```python
from build123d import *

# Parameters (mm, degrees)
SKETCH1_W           = 50.8
SKETCH1_H           = 25.4
SKETCH1_W_2         = 44.45
SKETCH1_H_2         = 19.05
BOSS_EXTRUDE1_DEPTH = 254
SKETCH2_R           = 14.2875
CUT_EXTRUDE1_DEPTH  = 26.4
SKETCH3_R           = 3.175
CUT_EXTRUDE2_DEPTH  = 26.4
CUT_EXTRUDE3_DEPTH  = 26.4


with BuildPart() as part:
    # Sketch1 → Boss-Extrude1 (new body)
    with BuildSketch(Plane.XY):
        with Locations((25.4, 12.7)):
            Rectangle(SKETCH1_W, SKETCH1_H)
        with Locations((25.4, 12.7)):
            Rectangle(SKETCH1_W_2, SKETCH1_H_2, mode=Mode.SUBTRACT)
    extrude(amount=BOSS_EXTRUDE1_DEPTH)

    # Sketch2 → Cut-Extrude1 (cut, through all)
    with BuildSketch(Plane(origin=(0, 25.4, 0), x_dir=(1, 0, 0), z_dir=(0, 1, 0))):
        with Locations((31.75, -19.05)):
            Circle(SKETCH2_R)
        with Locations((31.75, -171.45)):
            Circle(SKETCH2_R)
    extrude(amount=-CUT_EXTRUDE1_DEPTH, mode=Mode.SUBTRACT)

    # Sketch3 → Cut-Extrude2 (cut, through all)
    with BuildSketch(Plane(origin=(0, 25.4, 0), x_dir=(1, 0, 0), z_dir=(0, 1, 0))):
        with Locations((25.4, -244.475)):
            Circle(SKETCH3_R)
    extrude(amount=-CUT_EXTRUDE2_DEPTH, mode=Mode.SUBTRACT)

    # Sketch4 → Cut-Extrude3 (cut, through all)
    with BuildSketch(Plane(origin=(0, 25.4, 0), x_dir=(1, 0, 0), z_dir=(0, 1, 0))):
        with BuildLine():
            Line((36.358855328, -254), (36.358855328, -206.035443665))
            ThreePointArc((36.358855328, -206.035443665), (40.588568674, -195.824012339), (50.8, -191.594298992))
            Line((50.8, -191.594298992), (50.8, -254))
            Line((50.8, -254), (36.358855328, -254))
        make_face()
    extrude(amount=-CUT_EXTRUDE3_DEPTH, mode=Mode.SUBTRACT)


solid = part.part
```
Here's how the part is built. I have some questions about the finished solid (model axes, mm). A direction names the side the tool comes from. Give positions to 0.01 mm unless a question says otherwise; leave off trailing zeros. Loops run counter-clockwise (first coordinate to the right, second up) from the corner with the lowest first, then second, coordinate; pieces in that order, holes last. Notation, with made-up numbers: M 56,37 L 79,37 A21 cw 79,47 Z; hole C 13,63 d7. An arc over 180 degrees is marked long. Use one line per item in the form item = value. Start each with the question number.
Q1. If we section it at A-A (z = 171.45): Write out the boundary of the cut face in (x, y) (1 decimal), then the cut area to 3 significant figures.
Q2. Will this pin go through, and if not, where does the flat tip stop? pin 1 Ø3.5 at (y, z) = (24, 235) entering from +X.
Q3. If we section it at C-C (y = 10): Write out the boundary of the cut face in (x, z) (3 decimals), then the cut area to 3 significant figures.
Q4. Thinking about a two-plate mould opening in X: for faces 3 (the flat face through (25, 25.4, 125)), 4 (the cylindrical face through (24.712, 1.61, 247.574)), 5 (the flat face through (50.8, 13, 94)), which applies, +X half, -X half, draft (parallel to the pull), parting line (faces both ways), or undercut?
Q5. Which directions (+Z, -Z, +X, -X, +Y, -Y) give clear straight access to the entire face, cutting with the end or side of a thin tool? Please do faces 1 (the flat face through (25, 23, 0)), 2 (the flat face through (3.175, 13, 125)).
Q6. If we section it at B-B (x = 31.75): Write out the boundary of the cut face in (y, z) (1 decimal), then the cut area to 3 significant figures.
Q7. If we section it at D-D (x = 11): Write out the boundary of the cut face in (y, z) (3 decimals), then the cut area to 3 significant figures.
Q8. I need wall thicknesses on line 1 along Z through (x, y) = (31.75, 2.25); line 2 along Y through (x, z) = (19, 162) (3 decimals); line 3 along X through (y, z) = (2.15, 19.05). Which ranges of each line are inside material? Lowest first, please.
Taken from the geometry:
q1.outline = M 0,0 L 17.5,0 L 17.5,3.2 L 3.2,3.2 L 3.2,22.2 L 17.5,22.2 L 17.5,25.4 L 0,25.4 Z; M 46,0 L 50.8,0 L 50.8,25.4 L 46,25.4 L 46,22.2 L 47.6,22.2 L 47.6,3.2 L 46,3.2 Z
q1.area = 262 mm^2
q2.pin_1 = 36.36
q3.outline = M 0,0 L 3.175,0 L 3.175,254 L 0,254 Z; M 47.625,0 L 50.8,0 L 50.8,191.594 A14.441 cw 47.625,191.948 Z
q3.area = 1,420 mm^2
q4.face_3 = draft
q4.face_4 = undercut
q4.face_5 = +X half
q5.face_1 = -Z, +X, -X, +Y, -Y
q5.face_2 = +Z, -Z
q6.outline = M 0,0 L 3.2,0 L 3.2,4.8 L 0,4.8 Z; M 0,33.3 L 3.2,33.3 L 3.2,157.2 L 0,157.2 Z; M 0,185.7 L 3.2,185.7 L 3.2,254 L 0,254 Z; M 22.2,0 L 25.4,0 L 25.4,4.8 L 22.2,4.8 Z; M 22.2,33.3 L 25.4,33.3 L 25.4,157.2 L 22.2,157.2 Z; M 22.2,185.7 L 25.4,185.7 L 25.4,254 L 22.2,254 Z
q6.area = 1,250 mm^2
q7.outline = M 0,0 L 3.175,0 L 3.175,254 L 0,254 Z; M 22.225,0 L 25.4,0 L 25.4,254 L 22.225,254 Z
q7.area = 1,610 mm^2
q8.line_1 = 0 to 4.76, 33.34 to 157.16, 185.74 to 254
q8.line_2 = 0 to 3.175, 22.225 to 25.4
q8.line_3 = 0 to 17.46, 46.04 to 50.8
